Read the model definition and answer for the solid it produces. Units are mm, in the model's axes. Face numbers are marked on the shaded views. A direction names the side the tool comes from. Round coordinates to 2 decimals unless told otherwise and drop trailing zeros. Order: outer loops, then holes, each group sorted by start corner. A loop starts at its lowest first (then second) coordinate and runs counter-clockwise, first axis right, second up. Notation, with made-up numbers: (-7.5, 55) -> (37.5, 55) arc R16 cw to (37.5, 59) -> close; hole circle Ø7 at (-20, -9.75). An arc over 180 degrees is marked (long way). Use a Markdown table: item, result. Add a question column.
1. For the marked faces 1, 2 and 3, determine the directions among +Z, -Z, +X, -X, +Y, -Y from which every point of the face is accessible in a straight line to the end or side of a thin tool.
2. Section C-C, the plane x = 5 is taken. Give the vertices of the cut face in (y, z), then the cut area to 3 significant figures.
3. Given pin 1 (1.5 mm diameter, centred on x = 7.5, y = 6, fed in from -Z); pin 2 (2 mm diameter, centred on x = 6, y = 5.5, fed in from +Z); pin 3 (3 mm diameter, centred on x = 7, y = 3.5, fed in from -Z), each flat-ended and moving along its own axis, determine where each tip first touches the part or whether it passes through.
4. Consider L1, parallel to X at y = 5, z = -18; L2, parallel to X at y = 5, z = -7; L3, parallel to Y at x = 19, z = -13. Determine where each line is inside the solid, lowest interval first. Write a range as [from, to].
5. Section B-B, the plane y = 5 is taken. Give the vertices of the cut face in (x, z).
6. The mould has two halves that part along Y. Classify the marked faces 4, 5 and 6: +Y half, -Y half, draft (parallel to the pull), parting line (faces both ways), or undercut.
7. Section A-A, the plane z = -16 is taken. Give the vertices of the cut face in (x, y).
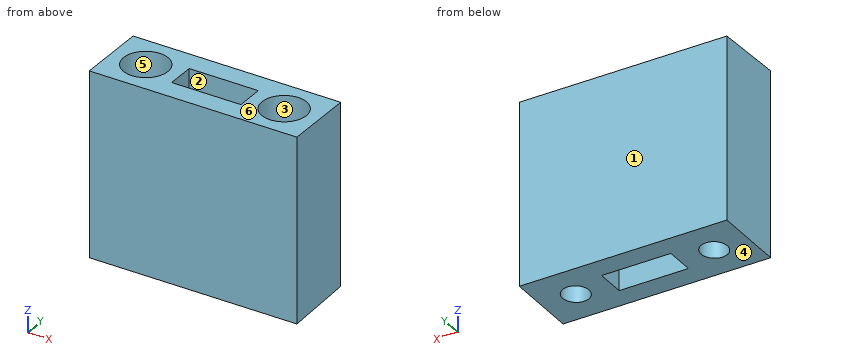
```python
from build123d import *

# Parameters (mm, degrees)
SKETCH_W     = 15
SKETCH_H     = 10
PAD_DEPTH    = 26
PAD001_DEPTH = 15
SKETCH005_W  = 10
SKETCH005_H  = 4
POCKET_DEPTH = 26.401


with BuildPart() as revolution:
    # Sketch004 → Revolution (revolve)
    with BuildSketch(Plane.YZ.offset(5)):
        Polygon((5, 0), (8.2, 0), (8.2, 10), (6.9, 11.3), (6.9, 27), (5, 27), align=None)
    revolve(axis=Axis((5, 5, 13.2), (0, 0, -1)))


with BuildPart() as pad:
    # Sketch → Pad (new body)
    with BuildSketch(Plane.XY):
        with Locations((7.5, 5)):
            Rectangle(SKETCH_W, SKETCH_H)
    extrude(amount=PAD_DEPTH)


with BuildPart() as pad001:
    # Pad001 base: copy of Pad
    add(pad.part)

    # Sketch001 → Pad001 (new body)
    with BuildSketch(Plane.YZ.offset(15)):
        Polygon((0, 26), (10, 26), (0, 26.4), align=None)
    extrude(amount=-PAD001_DEPTH)


with BuildPart() as cut:
    # Fusion base: copy of Pad
    add(pad.part)

    # Fusion: union Pad001
    add(pad001.part)

    # Cut: cut Revolution
    add(revolution.part, mode=Mode.SUBTRACT)


with BuildPart() as part_mirroring:
    # Part__Mirroring: instance of Cut
    add(cut.part.mirror(Plane(origin=(15, 0, 0), x_dir=(0, -1, 0), z_dir=(1, 0, 0))))


with BuildPart() as fusion001:
    # Fusion001 base: copy of Cut
    add(cut.part)

    # Fusion001: union Part__Mirroring
    add(part_mirroring.part)


with BuildPart() as pocket:
    # Part__Mirroring001: instance of Fusion001
    add(fusion001.part.mirror(Plane(origin=(0, 0, 0), x_dir=(0, 1, 0), z_dir=(0, 0, 1))))

    # Sketch005 → Pocket (cut, through all)
    with BuildSketch(Plane.XY):
        with Locations((15, 5)):
            Rectangle(SKETCH005_W, SKETCH005_H)
    extrude(amount=-POCKET_DEPTH, mode=Mode.SUBTRACT)


solid = pocket.part
```
Verdict:
| question | item | result |
|---|---|---|
| 1 | face 1 | +Z, -Z, +X, -X, +Y |
| 1 | face 2 | +Z, -Z |
| 1 | face 3 | +Z |
| 2 | outline | (0, -26.4) -> (3.1, -26.28) -> (3.1, -11.3) -> (1.8, -10) -> (1.8, 0) -> (0, 0) -> close; (6.9, -26.12) -> (10, -26) -> (10, 0) -> (8.2, 0) -> (8.2, -10) -> (6.9, -11.3) -> close |
| 2 | area | 135 mm2 |
| 3 | pin 1 | stops at z = -26.19 |
| 3 | pin 2 | stops at z = -11.08 |
| 3 | pin 3 | stops at z = -26.32 |
| 4 | L1 | x = [0, 3.1], [6.9, 10], [20, 23.1], [26.9, 30] |
| 4 | L2 | x = [0, 1.8], [8.2, 10], [20, 21.8], [28.2, 30] |
| 4 | L3 | y = [0, 3], [7, 10] |
| 5 | outline | (0, -26.2) -> (3.1, -26.2) -> (3.1, -11.3) -> (1.8, -10) -> (1.8, 0) -> (0, 0) -> close; (6.9, -26.2) -> (10, -26.2) -> (10, 0) -> (8.2, 0) -> (8.2, -10) -> (6.9, -11.3) -> close; (20, -26.2) -> (23.1, -26.2) -> (23.1, -11.3) -> (21.8, -10) -> (21.8, 0) -> (20, 0) -> close; (26.9, -26.2) -> (30, -26.2) -> (30, 0) -> (28.2, 0) -> (28.2, -10) -> (26.9, -11.3) -> close |
| 6 | face 4 | +Y half |
| 6 | face 5 | undercut |
| 6 | face 6 | draft |
| 7 | outline | (0, 0) -> (30, 0) -> (30, 10) -> (0, 10) -> close; hole circle Ø3.8 at (5, 5); hole (10, 3) -> (20, 3) -> (20, 7) -> (10, 7) -> close; hole circle Ø3.8 at (25, 5) |
